The figure shows three views and two pictorial views of one solid part (mm, origin at its lowest corner). Answer the questions. Give positions to 0.01 mm unless a question says otherwise; leave off trailing zeros. Loops run counter-clockwise (first coordinate to the right, second up) from the corner with the lowest first, then second, coordinate; pieces in that order, holes last.
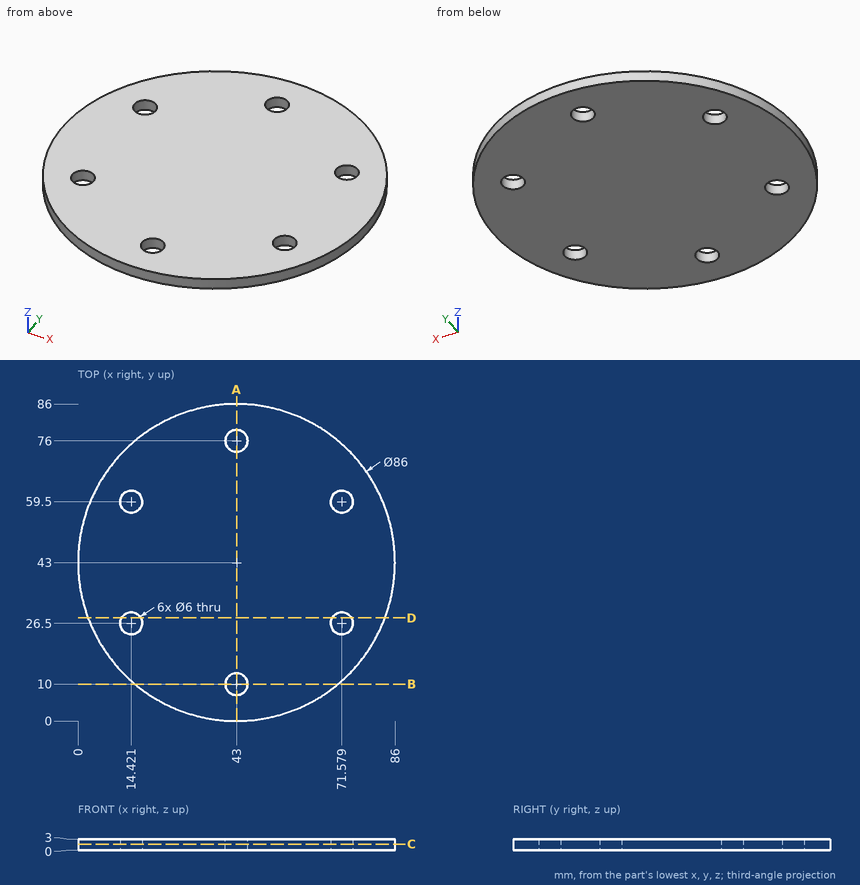
Q1. Section D-D on y = 28 is taken. Give the vertices of the cut face in (x, z), plus the area to 3 significant figures.
Q2. Consider line 1 along Y through (x, z) = (43, 1.2); line 2 along X through (y, z) = (59, 1.3); line 3 along X through (y, z) = (66.5, 1.75). Determine where each line is inside the solid, lowest interval first.
Q3. Given pin 1 (5.5 mm diameter, centred on x = 14.42, y = 59.5, fed in from -Z); pin 2 (1 mm diameter, centred on x = 29, z = 0.5, fed in from -Y), each flat-ended and moving along its own axis, determine where each tip first touches the part or whether it passes through.
Q4. Section C-C on z = 1.6 is taken. Give the vertices of the cut face in (x, y).
Q5. Section A-A on x = 43 is taken. Give the vertices of the cut face in (y, z).
Q6. Section B-B on y = 10 is taken. Give the vertices of the cut face in (x, z).
Check result:
1. outline: (2.7, 0) - (11.82, 0) - (11.82, 3) - (2.7, 3) - close; (17.02, 0) - (68.98, 0) - (68.98, 3) - (17.02, 3) - close; (74.18, 0) - (83.3, 0) - (83.3, 3) - (74.18, 3) - close
1. area: 211 mm2
2. line 1: y = 0 to 7, 13 to 73, 79 to 86
2. line 2: x = 3.09 to 11.46, 17.38 to 68.62, 74.54 to 82.91
2. line 3: x = 6.99 to 79.01
3. pin 1: passes through
3. pin 2: stops at y = 2.17
4. outline: circle Ø86 at (43, 43); hole circle Ø6 at (14.42, 26.5); hole circle Ø6 at (14.42, 59.5); hole circle Ø6 at (43, 10); hole circle Ø6 at (43, 76); hole circle Ø6 at (71.58, 26.5); hole circle Ø6 at (71.58, 59.5)
5. outline: (0, 0) - (7, 0) - (7, 3) - (0, 3) - close; (13, 0) - (73, 0) - (73, 3) - (13, 3) - close; (79, 0) - (86, 0) - (86, 3) - (79, 3) - close
6. outline: (15.43, 0) - (40, 0) - (40, 3) - (15.43, 3) - close; (46, 0) - (70.57, 0) - (70.57, 3) - (46, 3) - close
